```python
from build123d import *

# Parameters (mm, degrees)
SKETCH1_R           = 12.7
BOSS_EXTRUDE1_DEPTH = 5
SKETCH2_W           = 76.2
SKETCH2_H           = 7.5
BOSS_EXTRUDE2_DEPTH = 5
SKETCH3_R           = 12.7
BOSS_EXTRUDE3_DEPTH = 5
SKETCH4_R           = 9.525
CUT_EXTRUDE1_DEPTH  = 2.5
FILLET1_R           = 2.54


with BuildPart() as part:
    # Sketch1 → Boss-Extrude1 (new body)
    with BuildSketch(Plane(origin=(0, 0, 0), x_dir=(1, 0, 0), z_dir=(0, 1, 0))):
        with Locations(Location((0, 0, 0), (0, 0, 270))):
            Circle(SKETCH1_R)
    extrude(amount=BOSS_EXTRUDE1_DEPTH)

    # Sketch2 → Boss-Extrude2 (add)
    with BuildSketch(Plane(origin=(0, 5, 0), x_dir=(1, 0, 0), z_dir=(0, 1, 0))):
        Rectangle(SKETCH2_W, SKETCH2_H)
    extrude(amount=-BOSS_EXTRUDE2_DEPTH)

    # Sketch3 → Boss-Extrude3 (add)
    with BuildSketch(Plane(origin=(0, 5, 0), x_dir=(1, 0, 0), z_dir=(0, 1, 0))):
        with Locations((-33.819087464, 0)):
            Circle(SKETCH3_R)
    boss_extrude3 = extrude(amount=-BOSS_EXTRUDE3_DEPTH)

    # Sketch4 → Cut-Extrude1 (cut)
    with BuildSketch(Plane(origin=(0, 5, 0), x_dir=(1, 0, 0), z_dir=(0, 1, 0))):
        with Locations(Location((-33.819087464, 0, 0), (0, 0, 270))):
            Circle(SKETCH4_R)
    cut_extrude1 = extrude(amount=-CUT_EXTRUDE1_DEPTH, mode=Mode.SUBTRACT)

    # Mirror1: Boss-Extrude3, Cut-Extrude1 across plane
    add(boss_extrude3.mirror(Plane(origin=(0, 0, 0), x_dir=(0, 0, 1), z_dir=(1, 0, 0))))
    add(cut_extrude1.mirror(Plane(origin=(0, 0, 0), x_dir=(0, 0, 1), z_dir=(1, 0, 0))), mode=Mode.SUBTRACT)

    # Fillet1
    fillet1_edges = [part.edges().sort_by_distance(p)[0] for p in [
        (16.909543732, 0, -3.75),
        (-16.909543732, 0, 3.75),
        (-16.909543732, 0, -3.75),
        (16.909543732, 0, 3.75),
    ]]
    fillet(fillet1_edges, radius=FILLET1_R)


solid = part.part
```
Design review of the part built by this model. Coordinates are the model's own, in mm. A direction names the side the tool comes from. Give positions to 0.01 mm unless a question says otherwise; leave off trailing zeros. Order: outer loops, then holes, each group sorted by start corner. A loop starts at its lowest first (then second) coordinate and runs counter-clockwise, first axis right, second up. Notation, with made-up numbers: (21.25, 19.25) -> (43.25, 19.25) arc R22 cw to (43.25, 50.25) -> close; hole circle Ø7 at (24, 6). An arc over 180 degrees is marked (long way). Write item = value, one per line. Start each with the question number.
(1) We need section A-A on z = 5.5. Write out the cut boundary in (x, y), plus the area to 3 significant figures.
(2) For faces 1 (the face through (16.976, 0.764, 3.026)), 2 (the face through (17, 4, 3.75)), 3 (the face through (-17, 4, -3.75)), 4 (the face through (34, 2.5, 0)), 5 (the face through (-16.843, 0.764, -3.026)), list the 3-axis set-ups (+Z, -Z, +X, -X, +Y, -Y) from which the entire face can be reached by the end or side of a thin tool; tool diameter is ignored.
(3) We need section C-C on y = 4.2. Write out the cut boundary in (x, z) (3 decimals), plus the area to 3 significant figures.
(4) Mouldability with a two-part tool opening along Z and no side actions: class faces 6 (the face through (-16.843, 0.764, 3.026)), 7 (the face through (-24.375, 3.768, -1.24)), 8 (the face through (17, 4, -3.75)) as +Z half, -Z half, draft (parallel to the pull), parting line (faces both ways), or undercut.
(5) We need section B-B on x = 16. Write out the cut boundary in (y, z), plus the area to 3 significant figures.
(6) We need section D-D on z = 0. Write out the cut boundary in (x, y), plus the area to 3 significant figures.
(7) For pin 1 (1 mm diameter, centred on y = 2.5, z = 8, fed in from -X); pin 2 (1.5 mm diameter, centred on x = -8, y = 1, fed in from -Z); pin 3 (0.7 mm diameter, centred on x = 16.5, y = 4, fed in from -Z), all flat-tipped, find the tip position at first contact; note any pin that passes through.
(8) To check wall thickness, follow line 1 along X through (y, z) = (2.65, 2.75); line 2 along X through (y, z) = (2.35, -10.75); line 3 along X through (y, z) = (4, 5.75). State the ranges of each line that lie inside material, in increasing order.
Numbers:
q1.outline = (-45.27, 0) -> (-22.37, 0) -> (-22.37, 5) -> (-26.04, 5) -> (-26.04, 2.5) -> (-41.6, 2.5) -> (-41.6, 5) -> (-45.27, 5) -> close; (-11.45, 0) -> (11.45, 0) -> (11.45, 5) -> (-11.45, 5) -> close; (22.37, 0) -> (45.27, 0) -> (45.27, 5) -> (41.6, 5) -> (41.6, 2.5) -> (26.04, 2.5) -> (26.04, 5) -> (22.37, 5) -> close
q1.area = 266 mm^2
q2.face_1 = +Z, -Y
q2.face_2 = +Z, +Y, -Y
q2.face_3 = -Z, +Y, -Y
q2.face_4 = +Y
q2.face_5 = -Z, -Y
q3.outline = (-21.685, -3.75) -> (-12.134, -3.75) arc R12.7 ccw to (12.134, -3.75) -> (21.685, -3.75) arc R12.7 ccw (long way) to (21.685, 3.75) -> (12.134, 3.75) arc R12.7 ccw to (-12.134, 3.75) -> (-21.685, 3.75) arc R12.7 ccw (long way) to start; hole circle Ø19.05 at (-33.819, 0); hole circle Ø19.05 at (33.819, 0)
q3.area = 1,080 mm^2
q4.face_6 = +Z half
q4.face_7 = undercut
q4.face_8 = -Z half
q5.outline = (0, -1.21) arc R2.54 ccw to (2.54, -3.75) -> (5, -3.75) -> (5, 3.75) -> (2.54, 3.75) arc R2.54 ccw to (0, 1.21) -> close
q5.area = 34.7 mm^2
q6.outline = (-46.52, 0) -> (46.52, 0) -> (46.52, 5) -> (43.34, 5) -> (43.34, 2.5) -> (24.29, 2.5) -> (24.29, 5) -> (-24.29, 5) -> (-24.29, 2.5) -> (-43.34, 2.5) -> (-43.34, 5) -> (-46.52, 5) -> close
q6.area = 370 mm^2
q7.pin_1 = -44.07
q7.pin_2 = -10.43
q7.pin_3 = -3.75
q8.line_1 = -46.22 to -42.94, -24.7 to 24.7, 42.94 to 46.22
q8.line_2 = -40.58 to -27.06, -6.76 to 6.76, 27.06 to 40.58
q8.line_3 = -45.14 to -41.41, -26.23 to -22.5, -11.32 to 11.32, 22.5 to 26.23, 41.41 to 45.14
